Could you check a few things on this drawing? It's one solid part, dimensions in mm from its lowest x, y, z. A direction names the side the tool comes from. Round coordinates to 2 decimals unless told otherwise and drop trailing zeros. Loops run counter-clockwise (first coordinate to the right, second up) from the corner with the lowest first, then second, coordinate; pieces in that order, holes last. Notation, with made-up numbers: M 40,84 L 95,84 A24 ccw 95,107 Z; hole C -12.75,-34 d8. An arc over 180 degrees is marked long. Answer as CSV lines item,"result".
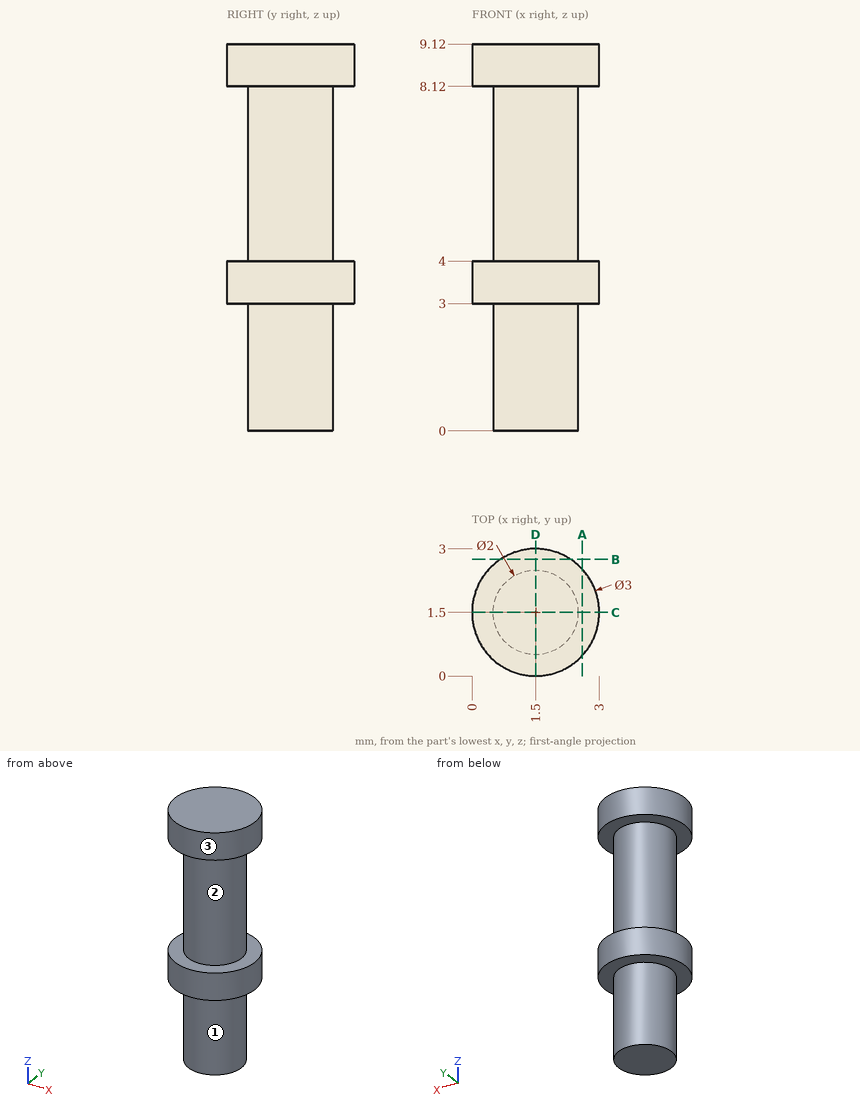
Item 1: If we section it at B-B on y = 2.75: Write out the boundary of the cut face in (x, z).
Output:
outline,"M 0.67,3 L 2.33,3 L 2.33,4 L 0.67,4 Z; M 0.67,8.12 L 2.33,8.12 L 2.33,9.12 L 0.67,9.12 Z"
Item 2: If I drill on line 1 along Z through (x, y) = (0.55, 0.8); line 2 along X through (y, z) = (1.65, 2.5); line 3 along Y through (x, z) = (0.85, 7), over which ranges is the centre line in solid material (lowest first)? Write a range as from..to.
Output:
line 1,"z = 3..4, 8.12..9.12"
line 2,"x = 0.51..2.49"
line 3,"y = 0.74..2.26"
Item 3: If we section it at A-A on x = 2.6: Write out the boundary of the cut face in (y, z).
Output:
outline,"M 0.48,3 L 2.52,3 L 2.52,4 L 0.48,4 Z; M 0.48,8.12 L 2.52,8.12 L 2.52,9.12 L 0.48,9.12 Z"
Item 4: Will this pin go through, and if not, where does the flat tip stop? pin 1 (1 mm diameter, centred on y = 1.5, z = 5.5, fed in from -X).
Output:
pin 1,"stops at x = 0.5"
Item 5: If we section it at C-C on y = 1.5: Write out the boundary of the cut face in (x, z), then the cut area to 3 significant figures.
Output:
outline,"M 0,3 L 0.5,3 L 0.5,0 L 2.5,0 L 2.5,3 L 3,3 L 3,4 L 2.5,4 L 2.5,8.12 L 3,8.12 L 3,9.12 L 0,9.12 L 0,8.12 L 0.5,8.12 L 0.5,4 L 0,4 Z"
area,"20.2 mm2"
Item 6: On a 3-axis mill with a long thin cutter (end or side, diameter ignored), from which of +Z, -Z, +X, -X, +Y, -Y can I reach the whole of each face in a straight line? I mean the marked faces 1, 2 and 3. Say none if no direction works.
Output:
face 1,"-Z"
face 2,"none"
face 3,"+Z, -Z"
